Autodesk Inventor part; units mm, degrees
ref_plane "YZ Plane" through (0, 0, 0) normal (1, 0, 0) x (0, 1, 0)
ref_plane "XZ Plane" through (0, 0, 0) normal (0, 1, 0) x (-1, 0, 0)
ref_plane "XY Plane" through (0, 0, 0) normal (0, 0, 1) x (1, 0, 0)
sketch "Sketch1" plane through (0, 0, 0) normal (0, 0, 1) x (1, 0, 0)
  line L0 (-25.4, 0) -> (-520.7, 0)
  line L1 (0, 25.4) -> (0, 406.4)
  line L2 (25.4, 406.4) -> (25.4, 0)
  line L3 (0, -25.4) -> (-520.7, -25.4)
  line L4 (-520.7, 0) -> (-520.7, -25.4)
  line L5 (25.4, 406.4) -> (0, 406.4)
  arc A0 (22.225, -25.4) -> (25.4, -22.225) centre (22.225, -22.225) ccw
  arc A1 (-25.4, 0) -> (0, 25.4) centre (-25.4, 25.4) ccw
  arc A2 (0, -25.4) -> (25.4, 0) centre (0, 0) ccw
  point P0 (0, 0)
  dimension "d0" = 520.7
  dimension "d1" = 406.4
  dimension "d2" = 25.4
  dimension "d3" = 3.175
  dimension "d6" = 25.4
extrude "Extrusion1" add sketch "Sketch1" along normal blind 546.1
sketch "Sketch2" plane through (-520.7, -25.4, 0) normal (0, -1, 0) x (1, 0, 0)
  line L0 (520.7, 0) -> (520.7, 546.1) construction
  line L1 (520.7, 273.05) -> (0, 273.05) construction
  line L2 (0, 0) -> (0, 546.1) construction
  line L3 (495.3, 546.1) -> (0, 546.1) construction
  line L4 (260.35, 546.1) -> (260.35, 0) construction
  line L5 (0, 0) -> (520.7, 0) construction
  line L6 (495.3, 546.1) -> (495.3, 527.05)
  line L7 (495.3, 0) -> (495.3, 546.1)
  line L8 (495.3, 527.05) -> (25.4, 527.05)
  line L9 (25.4, 527.05) -> (25.4, 546.1)
  line L10 (495.3, 546.1) -> (25.4, 546.1)
  line L11 (495.3, 0) -> (0, 0) construction
  line L12 (495.3, 0) -> (495.3, 19.05)
  line L13 (495.3, 19.05) -> (25.4, 19.05)
  line L14 (25.4, 19.05) -> (25.4, 0)
  line L15 (495.3, 0) -> (25.4, 0)
  point P0 (25.4, 536.575)
  point P1 (25.4, 9.525)
  dimension "d7" = 19.05
  dimension "d8" = 25.4
extrude "Extrusion2" add sketch "Sketch2" along normal blind 25.4
sketch "Sketch4" plane through (0, -25.4, 0) normal (0, -1, 0) x (1, 0, 0)
  line L0 (-25.4, 527.05) -> (-25.4, 546.1)
  line L1 (-25.4, 527.05) -> (0, 527.05)
  line L2 (0, 0) -> (0, 546.1)
  line L3 (-25.4, 546.1) -> (-495.3, 546.1)
  line L4 (0, 546.1) -> (-25.4, 546.1)
  line L5 (-25.4, 546.1) -> (-25.4, 527.05)
  line L6 (25.4, 0) -> (25.4, 546.1) construction
  line L7 (25.4, 273.05) -> (-520.7, 273.05) construction
  line L8 (-520.7, 0) -> (-520.7, 546.1) construction
  line L9 (-495.3, 0) -> (-25.4, 0) construction
  line L10 (-247.65, 0) -> (-247.65, 546.1) construction
  line L11 (-25.4, 19.05) -> (-25.4, 0)
  line L12 (-25.4, 19.05) -> (0, 19.05)
  line L13 (0, 0) -> (-25.4, 0)
  line L14 (-25.4, 0) -> (-25.4, 19.05)
  line L15 (-495.3, 546.1) -> (-520.7, 546.1)
  line L16 (-520.7, 527.05) -> (-495.3, 527.05)
  line L17 (-495.3, 527.05) -> (-495.3, 546.1)
  line L18 (-495.3, 0) -> (-495.3, 19.05)
  line L19 (-495.3, 19.05) -> (-520.7, 19.05)
  line L20 (-520.7, 0) -> (-495.3, 0)
  line L21 (-520.7, 0) -> (-495.3, 0)
  line L22 (-495.3, 0) -> (-495.3, 19.05)
  line L23 (-25.4, 546.1) -> (-25.4, 527.05)
  line L24 (0, 546.1) -> (0, 527.05)
  line L25 (-495.3, 546.1) -> (-495.3, 527.05)
  line L26 (-520.7, 527.05) -> (-520.7, 546.1)
  line L27 (-495.3, 19.05) -> (-495.3, 0)
  line L28 (-520.7, 0) -> (-520.7, 19.05)
extrude "Extrusion3" add sketch "Sketch4" along normal blind 431.8
properties part number "chair"
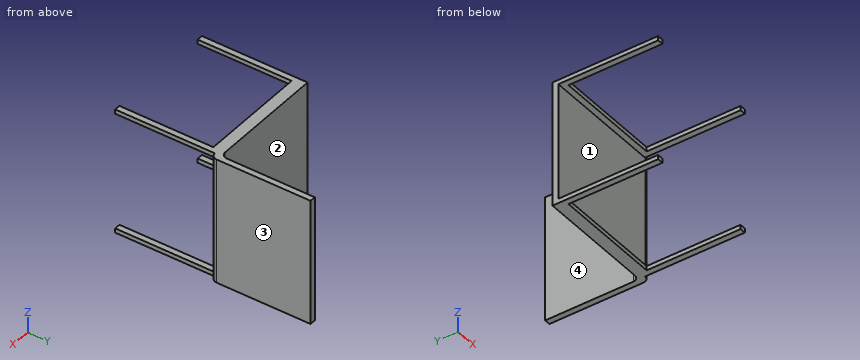
For this review, take the finished solid that the model builds, in its own axes (mm). Face numbers are marked on the shaded views. A direction names the side the tool comes from. Give positions to 0.01 mm unless a question says otherwise; leave off trailing zeros. Order: outer loops, then holes, each group sorted by start corner. A loop starts at its lowest first (then second) coordinate and runs counter-clockwise, first axis right, second up. Notation, with made-up numbers: (40.25, -9) - (98.25, -9) arc R27 ccw to (98.25, 30) - close; hole circle Ø7 at (30, 70.25). An arc over 180 degrees is marked (long way). Answer as a JSON object with one key per item and string values. Group by question number.
Item 1: Take a section at C-C on x = -293. Give the boundary of the cut face in (y, z), and give its area (3 significant figures).
Item 2: Machinability: for the marked faces 3 and 4, which of the approach directions +Z, -Z, +X, -X, +Y, -Y give a long, thin tool a straight path to every point of the face, cutting with its end or side? Answer none if there is none.
Item 3: Wall thickness on line 1 along Y through (x, z) = (-335.5, 142); line 2 along X through (y, z) = (44.5, 59); line 3 along Y through (x, z) = (-16, 262): over which ranges is each line inside the solid? List them lowest first.
Item 4: Clearance check with flat-ended pins moving along their axes: pin 1 Ø6 at (y, z) = (178, 368) entering from -X; pin 2 Ø15 at (x, z) = (-195, 532) entering from -Y; pin 3 Ø3 at (x, z) = (-263, 407.5) entering from -Y. State where each tip first meets the part, or that it passes through.
Item 5: Take a section at A-A on y = -151. Give the boundary of the cut face in (x, z).
Item 6: Take a section at D-D on y = 231.5. Give the boundary of the cut face in (x, z).
Item 7: Take a section at B-B on z = 63. Give the boundary of the cut face in (x, y), and give its area (3 significant figures).
Item 8: Draft analysis for pull direction Z (two halves, no side actions). For the marked faces 1 and 2, state which applies: pulls with the +Z half, pulls with the -Z half, needs draft (parallel to the pull), parting line crosses it, or undercut.
Reported:
{
 "1": {"outline": "(-50.8, 0) - (0, 0) - (0, 546.1) - (-50.8, 546.1) - (-50.8, 527.05) - (-25.4, 527.05) - (-25.4, 19.05) - (-50.8, 19.05) - close", "area": "14,800 mm^2"},
 "2": {"face 3": "+Z, -Z, +X, +Y, -Y", "face 4": "+Z, -Z, -X, +Y"},
 "3": {"line 1": "-25.4 to 0", "line 2": "0 to 25.4", "line 3": "-25.4 to 1.8"},
 "4": {"pin 1": "x = 0", "pin 2": "y = -50.8", "pin 3": "y = -25.4"},
 "5": {"outline": "(-520.7, 0) - (-495.3, 0) - (-495.3, 19.05) - (-520.7, 19.05) - close; (-520.7, 527.05) - (-495.3, 527.05) - (-495.3, 546.1) - (-520.7, 546.1) - close; (-25.4, 0) - (0, 0) - (0, 19.05) - (-25.4, 19.05) - close; (-25.4, 527.05) - (0, 527.05) - (0, 546.1) - (-25.4, 546.1) - close"},
 "6": {"outline": "(0, 0) - (25.4, 0) - (25.4, 546.1) - (0, 546.1) - close"},
 "7": {"outline": "(-520.7, -25.4) - (0, -25.4) arc R25.4 ccw to (25.4, 0) - (25.4, 406.4) - (0, 406.4) - (0, 25.4) arc R25.4 cw to (-25.4, 0) - (-520.7, 0) - close", "area": "24,200 mm^2"},
 "8": {"face 1": "undercut", "face 2": "needs draft"}
}
